```python
from build123d import *

# Parameters (mm, degrees)
SKETCH_1_W            = 230
SKETCH_1_H            = 400
SKETCH_1_R            = 2.5
EXTRUDE_1_DEPTH       = 3
SKETCH1_R             = 1.5
TOWER_HOLES_DEPTH     = 231.724944469
CUT_EXTRUDE2_DEPTH    = 7
SKETCH3_W             = 110
SKETCH3_H             = 110
CUT_EXTRUDE3_DEPTH    = 231.724944469
FILLET1_R             = 10
FILLET2_R             = 10
SKETCH4_W             = 200
SKETCH4_H             = 43
BOSS_EXTRUDE1_DEPTH   = 3
SKETCH5_R             = 1.5
CUT_EXTRUDE4_DEPTH    = 269.854979496
CUT_EXTRUDE5_DEPTH    = 269.854979496
FILLET3_R             = 10
FILLET4_R             = 2.5
SKETCH7_R             = 1.1
CUT_EXTRUDE6_DEPTH    = 269.854979496
SKETCH8_R             = 1.5
CUT_EXTRUDE7_DEPTH    = 269.854979496
SKETCH9_R             = 1.5
NUC_HOLES_DEPTH       = 269.854979496
SKETCH10_R            = 1.5
LIDAR_BOX_HOLES_DEPTH = 269.854979496


with BuildPart() as part:
    # Эскиз1 → Бобышка-Вытянуть1 (new body)
    with BuildSketch(Plane(origin=(0, 0, 0), x_dir=(1, 0, 0), z_dir=(0, 1, 0))):
        Rectangle(SKETCH_1_W, SKETCH_1_H)
        with Locations(Location((-60, -180, 0), (0, 0, 270))):
            Circle(SKETCH_1_R, mode=Mode.SUBTRACT)
        with Locations(Location((60, -180, 0), (0, 0, 90))):
            Circle(SKETCH_1_R, mode=Mode.SUBTRACT)
        with Locations(Location((60, -60, 0), (0, 0, 270))):
            Circle(SKETCH_1_R, mode=Mode.SUBTRACT)
        with Locations(Location((-60, -60, 0), (0, 0, 90))):
            Circle(SKETCH_1_R, mode=Mode.SUBTRACT)
        with Locations(Location((-60, 180, 0), (0, 0, 90))):
            Circle(SKETCH_1_R, mode=Mode.SUBTRACT)
        with Locations(Location((60, 180, 0), (0, 0, 270))):
            Circle(SKETCH_1_R, mode=Mode.SUBTRACT)
        with Locations(Location((60, 60, 0), (0, 0, 90))):
            Circle(SKETCH_1_R, mode=Mode.SUBTRACT)
        with Locations(Location((-60, 60, 0), (0, 0, 270))):
            Circle(SKETCH_1_R, mode=Mode.SUBTRACT)
    extrude(amount=EXTRUDE_1_DEPTH)

    # Sketch1 → Tower holes (cut, through all)
    with BuildSketch(Plane(origin=(0, 3, 0), x_dir=(1, 0, 0), z_dir=(0, 1, 0))):
        with Locations(Location((-105, 82.5, 0), (0, 0, 270))):
            Circle(SKETCH1_R)
        with Locations(Location((-105, 72.5, 0), (0, 0, 270))):
            Circle(SKETCH1_R)
        with Locations(Location((-82.5, 105, 0), (0, 0, 90))):
            Circle(SKETCH1_R)
        with Locations(Location((-72.5, 105, 0), (0, 0, 90))):
            Circle(SKETCH1_R)
        with Locations(Location((82.5, 105, 0), (0, 0, 270))):
            Circle(SKETCH1_R)
        with Locations(Location((72.5, 105, 0), (0, 0, 270))):
            Circle(SKETCH1_R)
        with Locations(Location((105, 82.5, 0), (0, 0, 90))):
            Circle(SKETCH1_R)
        with Locations(Location((105, 72.5, 0), (0, 0, 90))):
            Circle(SKETCH1_R)
        with Locations(Location((105, -82.5, 0), (0, 0, 270))):
            Circle(SKETCH1_R)
        with Locations(Location((105, -72.5, 0), (0, 0, 270))):
            Circle(SKETCH1_R)
        with Locations(Location((82.5, -105, 0), (0, 0, 90))):
            Circle(SKETCH1_R)
        with Locations(Location((72.5, -105, 0), (0, 0, 90))):
            Circle(SKETCH1_R)
        with Locations(Location((-82.5, -105, 0), (0, 0, 270))):
            Circle(SKETCH1_R)
        with Locations(Location((-72.5, -105, 0), (0, 0, 270))):
            Circle(SKETCH1_R)
        with Locations(Location((-105, -82.5, 0), (0, 0, 90))):
            Circle(SKETCH1_R)
        with Locations(Location((-105, -72.5, 0), (0, 0, 90))):
            Circle(SKETCH1_R)
        with Locations(Location((-105, 137.5, 0), (0, 0, 90))):
            Circle(SKETCH1_R)
        with Locations(Location((-105, 127.5, 0), (0, 0, 90))):
            Circle(SKETCH1_R)
        with Locations(Location((105, 127.5, 0), (0, 0, 270))):
            Circle(SKETCH1_R)
        with Locations(Location((105, 137.5, 0), (0, 0, 270))):
            Circle(SKETCH1_R)
        with Locations(Location((105, -127.5, 0), (0, 0, 90))):
            Circle(SKETCH1_R)
        with Locations(Location((105, -137.5, 0), (0, 0, 90))):
            Circle(SKETCH1_R)
        with Locations(Location((-105, -127.5, 0), (0, 0, 270))):
            Circle(SKETCH1_R)
        with Locations(Location((-105, -137.5, 0), (0, 0, 270))):
            Circle(SKETCH1_R)
    extrude(amount=-TOWER_HOLES_DEPTH, mode=Mode.SUBTRACT)

    # Sketch2 → Cut-Extrude2 (cut)
    with BuildSketch(Plane(origin=(0, 3, 0), x_dir=(1, 0, 0), z_dir=(0, 1, 0))):
        Polygon((-115, 200), (-70, 200), (-70, 155), (-110, 155), (-110, 105), (-115, 105), (-115, 155), align=None)
        Polygon((70, 200), (70, 155), (110, 155), (110, 105), (115, 105), (115, 155), (115, 200), align=None)
    extrude(amount=-CUT_EXTRUDE2_DEPTH, mode=Mode.SUBTRACT)

    # Sketch3 → Cut-Extrude3 (cut, through all)
    with BuildSketch(Plane(origin=(0, 3, 0), x_dir=(1, 0, 0), z_dir=(0, 1, 0))):
        with Locations((0, 120)):
            Rectangle(SKETCH3_W, SKETCH3_H)
    extrude(amount=-CUT_EXTRUDE3_DEPTH, mode=Mode.SUBTRACT)

    # Fillet1
    fillet1_edges = [part.edges().sort_by_distance(p)[0] for p in [
        (-55, 1.5, -65),
        (-55, 1.5, -175),
        (55, 1.5, -175),
        (55, 1.5, -65),
    ]]
    fillet(fillet1_edges, radius=FILLET1_R)

    # Fillet2
    fillet2_edges = [part.edges().sort_by_distance(p)[0] for p in [
        (70, 1.5, -200),
        (-70, 1.5, -200),
        (-70, 1.5, -155),
        (-110, 1.5, -155),
        (110, 1.5, -155),
        (70, 1.5, -155),
    ]]
    fillet(fillet2_edges, radius=FILLET2_R)

    # Sketch4 → Boss-Extrude1 (add)
    with BuildSketch(Plane(origin=(0, 0, 0), x_dir=(1, 0, 0), z_dir=(0, 1, 0))):
        with Locations((0, -221.5)):
            Rectangle(SKETCH4_W, SKETCH4_H)
    extrude(amount=BOSS_EXTRUDE1_DEPTH)

    # Sketch5 → Cut-Extrude4 (cut, through all)
    with BuildSketch(Plane(origin=(0, 3, 0), x_dir=(1, 0, 0), z_dir=(0, 1, 0))):
        with Locations(Location((26.5, -208, 0), (0, 0, 270))):
            Circle(SKETCH5_R)
        with Locations(Location((-26.5, -208, 0), (0, 0, 90))):
            Circle(SKETCH5_R)
        with Locations(Location((26.5, -234.5, 0), (0, 0, 270))):
            Circle(SKETCH5_R)
        with Locations(Location((-26.5, -234.5, 0), (0, 0, 90))):
            Circle(SKETCH5_R)
        with Locations(Location((26.5, -181.5, 0), (0, 0, 270))):
            Circle(SKETCH5_R)
        with Locations(Location((-26.5, -181.5, 0), (0, 0, 90))):
            Circle(SKETCH5_R)
        with Locations(Location((26.5, -155, 0), (0, 0, 270))):
            Circle(SKETCH5_R)
        with Locations(Location((-26.5, -155, 0), (0, 0, 90))):
            Circle(SKETCH5_R)
        with Locations(Location((26.5, -128.5, 0), (0, 0, 270))):
            Circle(SKETCH5_R)
        with Locations(Location((-26.5, -128.5, 0), (0, 0, 90))):
            Circle(SKETCH5_R)
        with Locations(Location((26.5, -102, 0), (0, 0, 270))):
            Circle(SKETCH5_R)
        with Locations(Location((-26.5, -102, 0), (0, 0, 90))):
            Circle(SKETCH5_R)
    extrude(amount=-CUT_EXTRUDE4_DEPTH, mode=Mode.SUBTRACT)

    # Sketch6 → Cut-Extrude5 (cut, through all)
    with BuildSketch(Plane(origin=(0, 3, 0), x_dir=(1, 0, 0), z_dir=(0, 1, 0))):
        Polygon((115, -160), (30, -243), (115, -243), align=None)
        Polygon((-115, -160), (-30, -243), (-115, -243), align=None)
    extrude(amount=-CUT_EXTRUDE5_DEPTH, mode=Mode.SUBTRACT)

    # Fillet3
    fillet3_edges = [part.edges().sort_by_distance(p)[0] for p in [
        (115, 1.5, 160),
        (30, 1.5, 243),
        (-30, 1.5, 243),
        (-115, 1.5, 160),
    ]]
    fillet(fillet3_edges, radius=FILLET3_R)

    # Fillet4
    fillet4_edges = [part.edges().sort_by_distance(p)[0] for p in [
        (110, 1.5, -105),
        (-110, 1.5, -105),
    ]]
    fillet(fillet4_edges, radius=FILLET4_R)
    fillet4_2_edges = [part.edges().sort_by_distance(p)[0] for p in [
        (115, 1.5, -105),
        (-115, 1.5, -105),
    ]]
    fillet(fillet4_2_edges, radius=FILLET4_R - 0.0001)  # a hair under: the kernel refuses the full size

    # Sketch7 → Cut-Extrude6 (cut, through all)
    with BuildSketch(Plane(origin=(0, 3, 0), x_dir=(1, 0, 0), z_dir=(0, 1, 0))):
        with Locations(Location((41.027426882, -190.3, 0), (0, 0, 270))):
            Circle(SKETCH7_R)
        with Locations(Location((48.013820265, -197.454740212, 0), (0, 0, 90))):
            Circle(SKETCH7_R)
        with Locations(Location((76.632781112, -169.509166679, 0), (0, 0, 270))):
            Circle(SKETCH7_R)
        with Locations(Location((69.646387729, -162.354426467, 0), (0, 0, 90))):
            Circle(SKETCH7_R)
        with Locations(Location((-69.646387729, -162.354426467, 0), (0, 0, 270))):
            Circle(SKETCH7_R)
        with Locations(Location((-76.632781112, -169.509166679, 0), (0, 0, 90))):
            Circle(SKETCH7_R)
        with Locations(Location((-48.013820265, -197.454740212, 0), (0, 0, 270))):
            Circle(SKETCH7_R)
        with Locations(Location((-41.027426882, -190.3, 0), (0, 0, 90))):
            Circle(SKETCH7_R)
    extrude(amount=-CUT_EXTRUDE6_DEPTH, mode=Mode.SUBTRACT)

    # Sketch8 → Cut-Extrude7 (cut, through all)
    with BuildSketch(Plane(origin=(0, 3, 0), x_dir=(1, 0, 0), z_dir=(0, 1, 0))):
        with Locations(Location((105, -32.5, 0), (0, 0, 270))):
            Circle(SKETCH8_R)
        with Locations(Location((105, -22.5, 0), (0, 0, 90))):
            Circle(SKETCH8_R)
        with Locations(Location((105, 22.5, 0), (0, 0, 270))):
            Circle(SKETCH8_R)
        with Locations(Location((105, 32.5, 0), (0, 0, 90))):
            Circle(SKETCH8_R)
        with Locations(Location((-105, 32.5, 0), (0, 0, 270))):
            Circle(SKETCH8_R)
        with Locations(Location((-105, 22.5, 0), (0, 0, 90))):
            Circle(SKETCH8_R)
        with Locations(Location((-105, -22.5, 0), (0, 0, 270))):
            Circle(SKETCH8_R)
        with Locations(Location((-105, -32.5, 0), (0, 0, 90))):
            Circle(SKETCH8_R)
    extrude(amount=-CUT_EXTRUDE7_DEPTH, mode=Mode.SUBTRACT)

    # Sketch9 → NUC holes (cut, through all)
    with BuildSketch(Plane(origin=(0, 3, 0), x_dir=(1, 0, 0), z_dir=(0, 1, 0))):
        with Locations(Location((40, 42.5, 0), (0, 0, 270))):
            Circle(SKETCH9_R)
        with Locations(Location((40, -42.5, 0), (0, 0, 90))):
            Circle(SKETCH9_R)
    extrude(amount=-NUC_HOLES_DEPTH, mode=Mode.SUBTRACT)

    # Sketch10 → Lidar box holes (cut, through all)
    with BuildSketch(Plane(origin=(0, 3, 0), x_dir=(1, 0, 0), z_dir=(0, 1, 0))):
        with Locations(Location((-96, 0, 0), (0, 0, 270))):
            Circle(SKETCH10_R)
        with Locations(Location((-24, 0, 0), (0, 0, 90))):
            Circle(SKETCH10_R)
    extrude(amount=-LIDAR_BOX_HOLES_DEPTH, mode=Mode.SUBTRACT)


solid = part.part
```
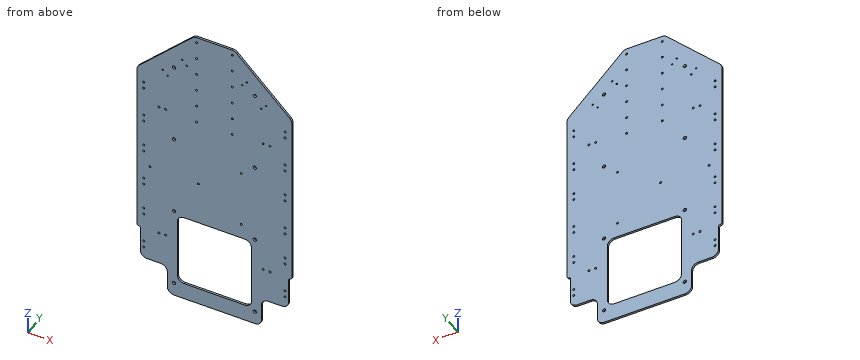
Check sheet for the modelled part. Datum: model origin and axes. Units: mm. Coordinates: 2 decimals unless noted, no trailing zeros. One line per question, with ' | ' between items. Start each with the question number.
Item 1: Gauge pin test, flat ends, axial feed: P1, Ø0.9, axis at x = 90.5, y = 1, coming from the -Z side; P2, Ø1.5, axis at y = 1, z = -129, coming from the -X side. Record the tip position at first contact, or that the pin passes through.
Item 2: Material ranges on line 1 (X direction, y = 0.6, z = 72.5); line 2 (X direction, y = 2.25, z = 0); line 3 (Z direction, x = 10, y = 2.65), recorded low to high.
Item 3: Sectioned sample at A-A on y = 2.3. Count the separate pieces of the cut face and the enclosed holes in it, and give its area (3 significant figures).
Answer below:
1) P1: stops at z = -155 | P2: stops at x = -110
2) line 1: x = -115 to -106.5, -103.5 to 103.5, 106.5 to 115 | line 2: x = -115 to -97.5, -94.5 to -25.5, -22.5 to 115 | line 3: z = -200 to -175, -65 to 243
3) separate pieces: 1 | enclosed holes: 65 | area: 77,700 mm^2
